Source: CAD feature listing. Evaluate the final solid. Frame: model axes, mm. A direction names the side the tool comes from. Coordinates: 2 decimals unless noted, no trailing zeros. Order: outer loops, then holes, each group sorted by start corner. A loop starts at its lowest first (then second) coordinate and runs counter-clockwise, first axis right, second up. Notation, with made-up numbers: (-11.5, 21.25) -> (30.5, 21.25) arc R26 ccw to (30.5, 50.25) -> close; hole circle Ø7 at (83.25, 65). An arc over 180 degrees is marked (long way). Write each question's results on one line, items separated by ' | '. Start each with the question number.
Autodesk Inventor part; units mm, degrees
ref_plane "YZ Plane" through (0, 0, 0) normal (1, 0, 0) x (0, 1, 0)
ref_plane "XZ Plane" through (0, 0, 0) normal (0, 1, 0) x (-1, 0, 0)
ref_plane "XY Plane" through (0, 0, 0) normal (0, 0, 1) x (1, 0, 0)
sketch "Эскиз1" plane through (0, 0, 0) normal (0, 1, 0) x (-1, 0, 0)
  circle A0 centre (0, 0) radius 12.5
  circle A1 centre (0, 0) radius 7.5
  dimension "d0" = 25
  dimension "d1" = 15
extrude "Выдавливание1" add sketch "Эскиз1" along normal blind 10
sketch "Эскиз2" plane through (0, 10, 0) normal (0, 1, 0) x (1, 0, 0)
  circle A0 centre (0, 0) radius 12.5
  line L0 (-2.1175, 12.3193) -> (0, 0)
  line L1 (2.1175, 12.3193) -> (0, 0)
  line L2 (-10.2084, 7.2138) -> (0, 0)
  line L3 (-7.2138, 10.2084) -> (0, 0)
  line L4 (-12.3193, -2.1175) -> (0, 0)
  line L5 (-12.3193, 2.1175) -> (0, 0)
  line L6 (-7.2138, -10.2084) -> (0, 0)
  line L7 (-10.2084, -7.2138) -> (0, 0)
  line L8 (2.1175, -12.3193) -> (0, 0)
  line L9 (-2.1175, -12.3193) -> (0, 0)
  line L10 (10.2084, -7.2138) -> (0, 0)
  line L11 (7.2138, -10.2084) -> (0, 0)
  line L12 (12.3193, 2.1175) -> (0, 0)
  line L13 (12.3193, -2.1175) -> (0, 0)
  line L14 (7.2138, 10.2084) -> (0, 0)
  line L15 (10.2084, 7.2138) -> (0, 0)
  dimension "d6" = 360
extrude "Выдавливание2" cut sketch "Эскиз2" against normal blind 3 contours A0 L13 L12 | L15 L14 A0 | L0 A0 L1 | L2 A0 L3 | L4 A0 L5 | L6 A0 L7 | L8 A0 L9 | L10 A0 L11
properties part number "pawn"
(1) Section A-A on z = 0. Return the cut outline in (x, y), then the cut area to 3 significant figures.
(2) Section D-D on x = -8.25. Return the cut outline in (y, z), then the cut area to 3 significant figures.
(3) Line query: L1, parallel to Y at x = 7.25, z = -6.25; L2, parallel to Z at x = 0, y = 6.75; L3, parallel to Z at x = 6, y = 4.5. Output: solid intervals per line, ascending.
(4) Section C-C on y = 9. Count the separate pieces of the cut face and the enclosed holes in it, then the cut area to 3 significant figures.
(5) Reachability of faces 1 (the cylindrical face through (-11.547, 3.819, 4.788)), 2 (the flat face through (0, 7, -10)), 3 (the flat face through (-1.7, 8.5, 9.9)), 4 (the flat face through (8.195, 8.521, 5.791)) from +Z, -Z, +X, -X, +Y, -Y: full face, straight path, thin tool, end or side. Return the list, or none.
(6) Section B-B on x = 0. Return the cut outline in (y, z), then the cut area to 3 significant figures.
(7) Draft query along X for faces 5 (the flat face through (-9.9, 8.5, -1.7)), 6 (the flat face through (-4, 10, -9)), 7 (the flat face through (7, 7, 7)), 8 (the flat face through (5.791, 8.521, -8.195)). Return one class per face: released by +X, released by -X, zero draft, split by the parting line, or undercut.
(8) First-contact query: P1, Ø3, axis at y = 6.5, z = 8.5, coming from the +X side; P2, Ø1, axis at x = -9.5, y = 6, coming from the +Z side; P3, Ø2, axis at x = 10.5, z = -0.5, coming from the +Y side. Flat tips, straight axial feed; report the tip coordinate or a pass-through.
Results list:
1) outline: (-12.5, 0) -> (-7.5, 0) -> (-7.5, 7) -> (-12.5, 7) -> close; (7.5, 0) -> (12.5, 0) -> (12.5, 7) -> (7.5, 7) -> close | area: 70.0 mm²
2) outline: (0, -9.39) -> (7, -9.39) -> (7, -5.83) -> (10, -5.83) -> (10, -1.42) -> (7, -1.42) -> (7, 1.42) -> (10, 1.42) -> (10, 5.83) -> (7, 5.83) -> (7, 9.39) -> (0, 9.39) -> close | area: 158 mm²
3) L1: y = 0 to 7 | L2: z = -12.5 to -7.5, 7.5 to 12.5 | L3: z = -10.97 to -4.5, 4.5 to 10.97
4) separate pieces: 8 | enclosed holes: 0 | area: 178 mm²
5) face 1: +Y, -Y | face 2: -Z, +Y | face 3: +Z, +Y | face 4: +Y
6) outline: (0, -12.5) -> (7, -12.5) -> (7, -7.5) -> (0, -7.5) -> close; (0, 7.5) -> (7, 7.5) -> (7, 12.5) -> (0, 12.5) -> close | area: 70.0 mm²
7) face 5: released by -X | face 6: zero draft | face 7: undercut | face 8: undercut
8) P1: stops at x = 10.36 | P2: stops at z = 8.67 | P3: stops at y = 7
